Verification items for the finished model (mm, model axes). A direction names the side the tool comes from. Round coordinates to 2 decimals unless told otherwise and drop trailing zeros. Order: outer loops, then holes, each group sorted by start corner. A loop starts at its lowest first (then second) coordinate and runs counter-clockwise, first axis right, second up. Notation, with made-up numbers: M 53.5,49 L 64.5,49 A18 ccw 64.5,68 Z; hole C 53,47.25 d4. An arc over 180 degrees is marked long. Answer as a JSON object with one key per item and string values. Group by question number.
```python
from build123d import *

# Parameters (mm, degrees)
SKETCH1_R           = 70
BOSS_EXTRUDE1_DEPTH = 1000
SKETCH3_W           = 36
SKETCH3_H           = 36
CUT_EXTRUDE1_DEPTH  = 100
EXTRUDE_THIN1_START = 50
SKETCH5_R           = 70
SKETCH5_R_2         = 69.9999
EXTRUDE_THIN1_DEPTH = 50


with BuildPart() as part:
    # Sketch1 → Boss-Extrude1 (new body)
    with BuildSketch(Plane.XY):
        Circle(SKETCH1_R)
    extrude(amount=-BOSS_EXTRUDE1_DEPTH)

    # Sketch3 → Cut-Extrude1 (cut)
    with BuildSketch(Plane.XY):
        with Locations((0, 60.4)):
            Rectangle(SKETCH3_W, SKETCH3_H)
    extrude(amount=-CUT_EXTRUDE1_DEPTH, mode=Mode.SUBTRACT)

    # Sketch5 → Extrude-Thin1 (add)
    with BuildSketch(Plane.XY.offset(-300).offset(EXTRUDE_THIN1_START)):
        Circle(SKETCH5_R)
        Circle(SKETCH5_R_2, mode=Mode.SUBTRACT)
    extrude(amount=-EXTRUDE_THIN1_DEPTH)


solid = part.part
```
Q1. Cross-section at C-C, the plane z = -670.5. Record the cut outline in (x, y).
Q2. Release check for a two-part mould opening along X. For faces 1 (the face through (-1, 0, 0)), 2 (the face through (18, 55, -49)), 3 (the face through (-15.175, -68.335, -493)) record: released by +X, released by -X, zero draft, split by the parting line, or undercut.
Q3. Thickness scan on line 1 (X direction, y = 61, z = -58.5); line 2 (Y direction, x = 3, z = -821); line 3 (X direction, y = 47.5, z = -365.5). Record the ranges inside material, lowest first. Write a range as from..to.
Q4. Tool access check on faces 4 (the face through (0, 42.4, -49)), 5 (the face through (-1, 1, -1000)). Record the directions out of +Z, -Z, +X, -X, +Y, -Y that give a thin tool (end or side, any length) a straight path to the whole face; none if there is none.
Q5. Gauge pin test, flat ends, axial feed: pin 1 Ø4 at (x, z) = (46, -639.5) entering from -Y; pin 2 Ø6 at (x, y) = (-7.5, 55) entering from +Z; pin 3 Ø20 at (y, z) = (61, -29) entering from -X. Record the tip position at first contact, or that the pin passes through.
Q6. Cross-section at D-D, the plane y = -55. Record the cut outline in (x, z).
Q7. Cross-section at A-A, the plane x = 0. Record the cut outline in (y, z), then the cut area to 3 significant figures.
Q8. Cross-section at B-B, the plane y = -19. Record the cut outline in (x, z).
Conclusion:
{
 "1": {"outline": "C 0,0 d140"},
 "2": {"face 1": "zero draft", "face 2": "undercut", "face 3": "split by the parting line"},
 "3": {"line 1": "-34.34..-18, 18..34.34", "line 2": "-69.94..69.94", "line 3": "-51.42..51.42"},
 "4": {"face 4": "+Z, +Y", "face 5": "-Z, +X, -X, +Y, -Y"},
 "5": {"pin 1": "y = -54.44", "pin 2": "z = -100", "pin 3": "x = -47.95"},
 "6": {"outline": "M -43.3,-1000 L 43.3,-1000 L 43.3,0 L -43.3,0 Z"},
 "7": {"outline": "M -70,-1000 L 70,-1000 L 70,-100 L 42.4,-100 L 42.4,0 L -70,0 Z", "area": "137,000 mm2"},
 "8": {"outline": "M -67.37,-1000 L 67.37,-1000 L 67.37,0 L -67.37,0 Z"}
}
